from build123d import *

# Parameters (mm, degrees)
SKETCH1_W               = 13
SKETCH1_H               = 8
BOSS_EXTRUDE1_DEPTH     = 3
CUT_EXTRUDE1_DEPTH      = 16.556349186
CUT_EXTRUDE1_DEPTH_BACK = 16.556349186
CUT_EXTRUDE2_DEPTH      = 16.556349186
CUT_EXTRUDE2_DEPTH_BACK = 16.556349186
SKETCH4_R               = 1.8
CUT_EXTRUDE3_DEPTH      = 0.8
SKETCH5_W               = 8
SKETCH5_H               = 1.1
BOSS_EXTRUDE2_DEPTH     = 2
FILLET1_R               = 4
CUT_EXTRUDE4_DEPTH      = 0.4


with BuildPart() as part:
    # Sketch1 → Boss-Extrude1 (new body)
    with BuildSketch(Plane(origin=(0, 0, 0), x_dir=(1, 0, 0), z_dir=(0, 1, 0))):
        with Locations((6.5, 4)):
            Rectangle(SKETCH1_W, SKETCH1_H)
    extrude(amount=BOSS_EXTRUDE1_DEPTH)

    # Sketch2 → Cut-Extrude1 (cut, two sides: drawn at the far end of the back side and taken through both)
    with BuildSketch(Plane.XY.offset(-CUT_EXTRUDE1_DEPTH_BACK)):
        Polygon((0, 0), (0.6, 3), (0, 3), align=None)
        Polygon((13, 0), (12.4, 3), (13, 3), align=None)
    extrude(amount=CUT_EXTRUDE1_DEPTH + CUT_EXTRUDE1_DEPTH_BACK, mode=Mode.SUBTRACT)

    # Sketch3 → Cut-Extrude2 (cut, two sides: drawn at the far end of the back side and taken through both)
    with BuildSketch(Plane(origin=(0, 0, 0), x_dir=(0, 0, -1), z_dir=(1, 0, 0)).offset(-CUT_EXTRUDE2_DEPTH_BACK)):
        Polygon((0, 0), (0.6, 3), (0, 3), align=None)
        Polygon((8, 3), (7.4, 3), (8, 0), align=None)
    extrude(amount=CUT_EXTRUDE2_DEPTH + CUT_EXTRUDE2_DEPTH_BACK, mode=Mode.SUBTRACT)

    # Sketch4 → Cut-Extrude3 (cut)
    with BuildSketch(Plane.XZ):
        with Locations(Location((6.50000125, -3.75, 0), (0, 0, 270))):
            Circle(SKETCH4_R)
    extrude(amount=-CUT_EXTRUDE3_DEPTH, mode=Mode.SUBTRACT)

    # Sketch5 → Boss-Extrude2 (add)
    with BuildSketch(Plane.XZ):
        with Locations((6.500011, -7.45)):
            Rectangle(SKETCH5_W, SKETCH5_H)
    extrude(amount=BOSS_EXTRUDE2_DEPTH)

    # Fillet1
    # the kernel refuses this fillet: 4 mm, written as the material it takes off along each edge
    with BuildSketch(Plane(origin=(10.500011, -2, -16.660254038), x_dir=(0, 1, 0), z_dir=(0, 0, 1)), Plane(origin=(2.500011, -2, 1.760254038), x_dir=(0, 1, 0), z_dir=(0, 0, -1))) as fillet1_piece_1:
        with BuildLine():
            CenterArc((4, 3.464101615), FILLET1_R, 180, 60)
            Line((0, 3.464101615), (-0.08, 3.464101615))
            Line((-0.08, 3.464101615), (-0.08, 0))
            Line((-0.08, 0), (0, -0.08))
            ThreePointArc((0, -0.08), (1, -0.08), (1.96, -0.069282032))
            Line((1.96, -0.069282032), (2, 0))
        make_face()
    extrude(amount=18.420508076, mode=Mode.SUBTRACT)

    # Sketch6 → Cut-Extrude4 (cut)
    # profile 1 of 3: a face of its own
    with BuildSketch(Plane(origin=(0, 3, 0), x_dir=(1, 0, 0), z_dir=(0, 1, 0))):
        Polygon((5.356583629, 2.605681315), (4.744804782, 2.605681315), (4.491799975, 3.297989008), (3.340357667, 3.297989008), (3.087352859, 2.605681315), (2.471968244, 2.605681315), (3.605982667, 5.605681315), (4.217160552, 5.605681315), align=None)
        Polygon((4.308506705, 3.797989008), (3.914275936, 4.874912084), (3.52124709, 3.797989008), align=None, mode=Mode.SUBTRACT)
    # profile 2 of 3: a face of its own
    with BuildSketch(Plane(origin=(0, 3, 0), x_dir=(1, 0, 0), z_dir=(0, 1, 0))):
        Polygon((5.664275936, 2.605681315), (5.664275936, 5.605681315), (6.241199013, 5.605681315), (6.241199013, 3.105681315), (7.779660552, 3.105681315), (7.779660552, 2.605681315), align=None)
    # profile 3 of 3: a face of its own
    with BuildSketch(Plane(origin=(0, 3, 0), x_dir=(1, 0, 0), z_dir=(0, 1, 0))):
        Polygon((8.895045167, 2.605681315), (8.895045167, 5.105681315), (8.010429782, 5.105681315), (8.010429782, 5.605681315), (10.356583629, 5.605681315), (10.356583629, 5.105681315), (9.471968244, 5.105681315), (9.471968244, 2.605681315), align=None)
    extrude(amount=-CUT_EXTRUDE4_DEPTH, mode=Mode.SUBTRACT)


solid = part.part
Can you work these out from the model? Positions are in its coordinate system, mm. A direction names the side the tool comes from. Coordinates: 2 decimals unless noted, no trailing zeros. Write each loop counter-clockwise with the first axis right and the second up, starting at its lowest first coordinate (ties: lowest second). Pieces come first, ordered by that corner, then holes. Notation, with made-up numbers: (47, 49.25) -> (63, 49.25) arc R24 ccw to (63, 84.25) -> close; hole circle Ø4 at (-16, 65). An arc over 180 degrees is marked (long way). Write each question's results on one line, items separated by ' | '. Start each with the question number.
Item 1: Please list where these lines run through material, in increasing order: probe 1 along Y at (x, z) = (3.5, -5); probe 2 along Y at (x, z) = (10.75, -6.5); probe 3 along X at (y, z) = (0.35, -3.75).
Item 2: If we section it at D-D, the plane z = -0.25: Write out the boundary of the cut face in (x, y).
Item 3: Thinking about a two-plate mould opening in Z: for faces 6 (the flat face through (12.7, 1.5, -4.1)), 7 (the flat face through (6, 2.6, -4)), 8 (the flat face through (6.4, 1.5, -7.7)), which applies, released by +Z, released by -Z, zero draft, split by the parting line, or undercut?
Item 4: If we section it at C-C, the plane y = -0.4: Write out the boundary of the cut face in (x, z), and give its area (3 significant figures).
Item 5: If we section it at A-A, the plane z = -4.25: Write out the boundary of the cut face in (x, y).
Item 6: On a 3-axis mill with a long thin cutter (end or side, diameter ignored), from which of +Z, -Z, +X, -X, +Y, -Y can I reach the whole of each face in a straight line? I mean faces 1 (the flat face through (6.5, -2, -7.4)), 2 (the flat face through (0.3, 1.5, -4.1)), 3 (the cylindrical face through (5.811, 0.394, -5.413)), 4 (the flat face through (4.779, 2.803, -4.127)), 5 (the flat face through (6, -1, -6.9)). Say none if no direction works.
Item 7: If we section it at B-B, the plane x = 5.5: Write out the boundary of the cut face in (y, z).
Item 8: I'm going to push flat-ended pins straight in: P1, Ø4, axis at x = 2.5, z = -6, coming from the -Y side; P2, Ø2.5, axis at x = 4.5, z = -5.5, coming from the -Y side; P3, Ø0.6, axis at x = 5, y = -1.5, coming from the +Z side. Where does each tip first touch, or does it pass through?
Answer block:
1) probe 1: 0 to 2.6 | probe 2: 0 to 3 | probe 3: 0.07 to 4.7, 8.3 to 12.93
2) outline: (0, 0) -> (13, 0) -> (12.75, 1.25) -> (0.25, 1.25) -> close
3) face 6: zero draft | face 7: undercut | face 8: released by -Z
4) outline: (2.76, -8) -> (10.24, -8) -> (10.24, -6.9) -> (2.76, -6.9) -> close | area: 8.22 mm²
5) outline: (0, 0) -> (4.77, 0) -> (4.77, 0.8) -> (8.23, 0.8) -> (8.23, 0) -> (13, 0) -> (12.4, 3) -> (9.47, 3) -> (9.47, 2.6) -> (8.9, 2.6) -> (8.9, 3) -> (6.24, 3) -> (6.24, 2.6) -> (5.66, 2.6) -> (5.66, 3) -> (4.73, 3) -> (4.73, 2.6) -> (4.14, 2.6) -> (4.14, 3) -> (3.69, 3) -> (3.69, 2.6) -> (3.09, 2.6) -> (3.09, 3) -> (0.6, 3) -> close
6) face 1: +Z, -Z, +X, -X, -Y | face 2: +Z, -Z, -X, +Y | face 3: -Y | face 4: +Y | face 5: +Z, +X, -X, -Y
7) outline: (-1.97, -8) -> (0, -8) -> (3, -7.4) -> (3, -0.6) -> (0, 0) -> (0, -2.25) -> (0.8, -2.25) -> (0.8, -5.25) -> (0, -5.25) -> (0, -6.9) -> (-1.97, -6.9) -> close
8) P1: y = -1.63 | P2: y = 0 | P3: z = -6.9
